from build123d import *

# Parameters (mm, degrees)
SKETCH_1_W          = 91
SKETCH_1_H          = 50
SKETCH_1_W_2        = 83
SKETCH_1_H_2        = 36
EXTRUDE_1_DEPTH     = 3
SKETCH_2_R          = 1.5
CUT_EXTRUDE_1_DEPTH = 3
SKETCH_3_R          = 1.6
CUT_EXTRUDE_2_DEPTH = 3
FILLET_1_R          = 4
SKETCH_4_W          = 30
SKETCH_4_H          = 35
EXTRUDE_2_DEPTH     = 3
SKETCH_5_R          = 1.25
CUT_EXTRUDE_3_DEPTH = 10
FILLET_2_R          = 3
SKETCH_6_W          = 18
SKETCH_6_H          = 27
CUT_EXTRUDE_4_DEPTH = 10
FILLET_3_R          = 2
SKETCH_7_W          = 38
SKETCH_7_H          = 10
SKETCH_7_R          = 1.6
EXTRUDE_3_DEPTH     = 3
FILLET_4_R          = 2
FILLET_5_R          = 2
SKETCH_8_W          = 30
SKETCH_8_H          = 41
CUT_EXTRUDE_5_DEPTH = 10


with BuildPart() as part:
    # 草图1 → 凸台-拉伸1 (new body)
    with BuildSketch(Plane.XY):
        Rectangle(SKETCH_1_W, SKETCH_1_H)
        Rectangle(SKETCH_1_W_2, SKETCH_1_H_2, mode=Mode.SUBTRACT)
    extrude(amount=EXTRUDE_1_DEPTH)

    # 草图2 → 切除-拉伸1 (cut)
    with BuildSketch(Plane.XY.offset(3)):
        with Locations((31.5, 21)):
            Circle(SKETCH_2_R)
        with Locations((31.5, -21)):
            Circle(SKETCH_2_R)
        with Locations((-31.5, -21)):
            Circle(SKETCH_2_R)
        with Locations((-31.5, 21)):
            Circle(SKETCH_2_R)
    extrude(amount=-CUT_EXTRUDE_1_DEPTH, mode=Mode.SUBTRACT)

    # 草图3 → 切除-拉伸2 (cut)
    with BuildSketch(Plane.XY.offset(3)):
        with Locations((41.5, 20)):
            Circle(SKETCH_3_R)
        with Locations((41.5, -20)):
            Circle(SKETCH_3_R)
        with Locations((-41.5, -20)):
            Circle(SKETCH_3_R)
        with Locations((-41.5, 20)):
            Circle(SKETCH_3_R)
    extrude(amount=-CUT_EXTRUDE_2_DEPTH, mode=Mode.SUBTRACT)

    # 圆角1
    fillet_1_edges = [part.edges().sort_by_distance(p)[0] for p in [
        (41.5, -18, 1.5),
        (41.5, 18, 1.5),
        (-41.5, 18, 1.5),
        (-41.5, -18, 1.5),
        (45.5, -25, 1.5),
        (-45.5, -25, 1.5),
        (-45.5, 25, 1.5),
        (45.5, 25, 1.5),
    ]]
    fillet(fillet_1_edges, radius=FILLET_1_R)

    # 草图4 → 凸台-拉伸2 (add)
    with BuildSketch(Plane(origin=(0, 0, 0), x_dir=(-1, 0, 0), z_dir=(0, 0, -1))):
        with Locations((-60.5, 0)):
            Rectangle(SKETCH_4_W, SKETCH_4_H)
    extrude(amount=-EXTRUDE_2_DEPTH)

    # 草图5 → 切除-拉伸3 (cut)
    with BuildSketch(Plane(origin=(0, 0, 0), x_dir=(-1, 0, 0), z_dir=(0, 0, -1))):
        with Locations((-70.5, -12)):
            Circle(SKETCH_5_R)
        with Locations((-70.5, 12)):
            Circle(SKETCH_5_R)
    extrude(amount=-CUT_EXTRUDE_3_DEPTH, mode=Mode.SUBTRACT)

    # 圆角2
    fillet_2_edges = [part.edges().sort_by_distance(p)[0] for p in [
        (45.5, 17.5, 1.5),
        (45.5, -17.5, 1.5),
        (75.5, -17.5, 1.5),
        (75.5, 17.5, 1.5),
    ]]
    fillet(fillet_2_edges, radius=FILLET_2_R)

    # 草图6 → 切除-拉伸4 (cut)
    with BuildSketch(Plane(origin=(0, 0, 0), x_dir=(-1, 0, 0), z_dir=(0, 0, -1))):
        with Locations((-57.5, 0)):
            Rectangle(SKETCH_6_W, SKETCH_6_H)
    extrude(amount=-CUT_EXTRUDE_4_DEPTH, mode=Mode.SUBTRACT)

    # 圆角3
    fillet_3_edges = [part.edges().sort_by_distance(p)[0] for p in [
        (66.5, -13.5, 1.5),
        (66.5, 13.5, 1.5),
        (48.5, 13.5, 1.5),
        (48.5, -13.5, 1.5),
    ]]
    fillet(fillet_3_edges, radius=FILLET_3_R)

    # 草图7 → 凸台-拉伸3 (add)
    # profile 1 of 2: a face of its own
    with BuildSketch(Plane(origin=(0, 0, 0), x_dir=(-1, 0, 0), z_dir=(0, 0, -1))):
        with Locations((0, 30)):
            Rectangle(SKETCH_7_W, SKETCH_7_H)
        with Locations((-16, 32)):
            Circle(SKETCH_7_R, mode=Mode.SUBTRACT)
        with Locations((16, 32)):
            Circle(SKETCH_7_R, mode=Mode.SUBTRACT)
    # profile 2 of 2: a face of its own
    with BuildSketch(Plane(origin=(0, 0, 0), x_dir=(-1, 0, 0), z_dir=(0, 0, -1))):
        with Locations((0, -30)):
            Rectangle(SKETCH_7_W, SKETCH_7_H)
        with Locations((16, -32)):
            Circle(SKETCH_7_R, mode=Mode.SUBTRACT)
        with Locations((-16, -32)):
            Circle(SKETCH_7_R, mode=Mode.SUBTRACT)
    extrude(amount=-EXTRUDE_3_DEPTH)

    # 圆角4
    fillet_4_edges = [part.edges().sort_by_distance(p)[0] for p in [
        (19, 35, 1.5),
        (-19, 35, 1.5),
        (-19, -35, 1.5),
        (19, -35, 1.5),
    ]]
    fillet(fillet_4_edges, radius=FILLET_4_R)

    # 圆角5
    fillet_5_edges = [part.edges().sort_by_distance(p)[0] for p in [
        (19, 25, 1.5),
        (-19, 25, 1.5),
        (-19, -25, 1.5),
        (19, -25, 1.5),
    ]]
    fillet(fillet_5_edges, radius=FILLET_5_R)

    # 草图8 → 切除-拉伸5 (cut)
    with BuildSketch(Plane.XY.offset(3)):
        with Locations((60.5, 0)):
            Rectangle(SKETCH_8_W, SKETCH_8_H)
    extrude(amount=-CUT_EXTRUDE_5_DEPTH, mode=Mode.SUBTRACT)


solid = part.part
The listing builds one solid part. Answer for the finished solid, in the listing's coordinates (mm). A direction names the side the tool comes from. Round coordinates to 2 decimals unless told otherwise and drop trailing zeros. Write each loop counter-clockwise with the first axis right and the second up, starting at its lowest first coordinate (ties: lowest second). Pieces come first, ordered by that corner, then holes. Notation, with made-up numbers: M 80,65 L 127,65 A27 ccw 127,93 Z; hole C -29,42.25 d2. An arc over 180 degrees is marked long. Write each question's results on one line, items separated by ' | '. Start each with the question number.
(1) Find the intervals of material crossed by line 1 (Y direction, x = -16, z = 0.9); line 2 (Y direction, x = 31.5, z = 1.7); line 3 (Y direction, x = 0.5, z = 2.4), in increasing order.
(2) For faces 4 (the cylindrical face through (-44.359, 23.797, 1.521)), 5 (the cylindrical face through (40.297, -16.859, 1.521)), 6 (the flat face through (-31, -25, 1)), determine the directions among +Z, -Z, +X, -X, +Y, -Y from which every point of the face is accessible in a straight line to the end or side of a thin tool.
(3) The part is cut by section A-A, the plane y = 4. Write down the section's boundary in (x, z), and give its area (3 significant figures).
(4) Determine the mould class of faces 1 (the flat face through (-1, 18, 1)), 2 (the flat face through (19, -30, 1)), 3 (the cylindrical face through (18.43, 34.4, 1.52)) for opening direction Y: +Y half, -Y half, draft (parallel to the pull), parting line (faces both ways), or undercut.
(5) The part is cut by section C-C, the plane x = 27. Write down the section's boundary in (y, z).
(6) Each of these flat-tipped pins is pushed along its axis until it touches: P1, Ø0.9, axis at y = 31.5, z = 1, coming from the +X side; P2, Ø1.5, axis at x = 36, z = 1.5, coming from the +Y side; P3, Ø1.5, axis at x = 18, z = 2.5, coming from the -Y side. Where does it stop, or does it pass through?
(7) The part is cut by section D-D, the plane z = 2.4. Give the number of separate pieces and of enclosed holes in the cut face, and give its area (3 significant figures).
(8) The part is cut by section B-B, the plane x = 16. Write down the section's boundary in (y, z).
Worked answers:
1) line 1: y = -35 to -33.6, -30.4 to -18, 18 to 30.4, 33.6 to 35 | line 2: y = -25 to -22.5, -19.5 to -18, 18 to 19.5, 22.5 to 25 | line 3: y = -35 to -18, 18 to 35
2) face 4: +Z, -Z, -X, +Y | face 5: +Z, -Z | face 6: +Z, -Z, -X, -Y
3) outline: M -45.5,0 L -41.5,0 L -41.5,3 L -45.5,3 Z; M 41.5,0 L 45.5,0 L 45.5,3 L 41.5,3 Z | area: 24.0 mm²
4) face 1: undercut | face 2: draft | face 3: +Y half
5) outline: M -25,0 L -18,0 L -18,3 L -25,3 Z; M 18,0 L 25,0 L 25,3 L 18,3 Z
6) P1: stops at x = 19 | P2: stops at y = 25 | P3: stops at y = -34.98
7) separate pieces: 1 | enclosed holes: 13 | area: 2,230 mm²
8) outline: M -35,0 L -33.6,0 L -33.6,3 L -35,3 Z; M -30.4,0 L -18,0 L -18,3 L -30.4,3 Z; M 18,0 L 30.4,0 L 30.4,3 L 18,3 Z; M 33.6,0 L 35,0 L 35,3 L 33.6,3 Z
